Verification items for the finished model (mm, model axes). A direction names the side the tool comes from. Give positions to 0.01 mm unless a question says otherwise; leave off trailing zeros. Write each loop counter-clockwise with the first axis right and the second up, starting at its lowest first coordinate (ties: lowest second). Pieces come first, ordered by that corner, then holes. Notation, with made-up numbers: (-33.75, 31) - (24.25, 31) arc R16 cw to (24.25, 52) - close; hole circle Ø2 at (-27, 18). An arc over 180 degrees is marked (long way). Put each result on its own line as item: value.
from build123d import *

# Parameters (mm, degrees)
SKETCH2_W           = 66.5
SKETCH2_H           = 63.5
BOSS_EXTRUDE1_DEPTH = 3
SKETCH6_W           = 72
SKETCH6_H           = 69
SKETCH6_W_2         = 66.5
SKETCH6_H_2         = 63.5
BOSS_EXTRUDE2_DEPTH = 5
SKETCH14_W          = 7.5
SKETCH14_H          = 59
BOSS_EXTRUDE4_DEPTH = 14
BOSS_EXTRUDE5_DEPTH = 1.5
SKETCH16_R          = 5.5
SKETCH16_R_2        = 2.5
BOSS_EXTRUDE6_DEPTH = 2
BOSS_EXTRUDE7_DEPTH = 10
BOSS_EXTRUDE8_DEPTH = 5
SKETCH19_W          = 15
SKETCH19_H          = 7
BOSS_EXTRUDE9_DEPTH = 3


with BuildPart() as part:
    # Sketch2 → Boss-Extrude1 (new body)
    with BuildSketch(Plane(origin=(0, 0, 0), x_dir=(1, 0, 0), z_dir=(0, 1, 0))):
        Rectangle(SKETCH2_W, SKETCH2_H)
    extrude(amount=BOSS_EXTRUDE1_DEPTH)

    # Sketch6 → Boss-Extrude2 (add)
    with BuildSketch(Plane(origin=(0, 0, 0), x_dir=(1, 0, 0), z_dir=(0, 1, 0))):
        Rectangle(SKETCH6_W, SKETCH6_H)
        Rectangle(SKETCH6_W_2, SKETCH6_H_2, mode=Mode.SUBTRACT)
    extrude(amount=BOSS_EXTRUDE2_DEPTH)

    # Sketch14 → Boss-Extrude4 (add)
    with BuildSketch(Plane(origin=(0, 3, 0), x_dir=(1, 0, 0), z_dir=(0, 1, 0))):
        with Locations((-32.25, -0.25)):
            Rectangle(SKETCH14_W, SKETCH14_H)
    extrude(amount=BOSS_EXTRUDE4_DEPTH)

    # Sketch15 → Boss-Extrude5 (add)
    with BuildSketch(Plane(origin=(0, 5, 0), x_dir=(1, 0, 0), z_dir=(0, 1, 0))):
        Polygon((-34.45, 32.95), (34.45, 32.95), (34.45, -32.95), (-34.45, -32.95), (-34.45, -29.75), (-36, -29.75), (-36, -34.5), (36, -34.5), (36, 34.5), (-36, 34.5), (-36, 29.25), (-34.45, 29.25), align=None)
    extrude(amount=BOSS_EXTRUDE5_DEPTH)

    # Sketch16 → Boss-Extrude6 (add)
    # profile 1 of 4: a face of its own
    with BuildSketch(Plane.XZ):
        with Locations((-38.75, 37.25)):
            Circle(SKETCH16_R)
        with Locations(Location((-38.75, 37.25, 0), (0, 0, 270))):
            Circle(SKETCH16_R_2, mode=Mode.SUBTRACT)
    # profile 2 of 4: a face of its own
    with BuildSketch(Plane.XZ):
        with Locations((38.75, 37.25)):
            Circle(SKETCH16_R)
        with Locations(Location((38.75, 37.25, 0), (0, 0, 270))):
            Circle(SKETCH16_R_2, mode=Mode.SUBTRACT)
    # profile 3 of 4: a face of its own
    with BuildSketch(Plane.XZ):
        with Locations((38.75, -37.25)):
            Circle(SKETCH16_R)
        with Locations(Location((38.75, -37.25, 0), (0, 0, 270))):
            Circle(SKETCH16_R_2, mode=Mode.SUBTRACT)
    # profile 4 of 4: a face of its own
    with BuildSketch(Plane.XZ):
        with Locations((-38.75, -37.25)):
            Circle(SKETCH16_R)
        with Locations(Location((-38.75, -37.25, 0), (0, 0, 270))):
            Circle(SKETCH16_R_2, mode=Mode.SUBTRACT)
    extrude(amount=-BOSS_EXTRUDE6_DEPTH)

    # Sketch17 → Boss-Extrude7 (add)
    with BuildSketch(Plane.ZY.offset(24)):
        Polygon((34.5, 6.5), (33.15, 6.5), (33.15, 8.35), (32.15, 8.35), (32.15, 8.75), (33.15, 10), (34.5, 10), align=None)
    boss_extrude7 = extrude(amount=-BOSS_EXTRUDE7_DEPTH)

    # Mirror1: Boss-Extrude7 across plane
    add(boss_extrude7.mirror(Plane.XY))

    # Sketch18 → Boss-Extrude8 (add, symmetric)
    with BuildSketch(Plane.XY):
        Polygon((36, 6.5), (34.65, 6.5), (34.65, 8.45), (33.65, 8.45), (33.65, 8.85), (34.90023603, 10), (36, 10), align=None)
    extrude(amount=BOSS_EXTRUDE8_DEPTH, both=True)

    # Sketch19 → Boss-Extrude9 (add)
    with BuildSketch(Plane(origin=(0, 3, 0), x_dir=(1, 0, 0), z_dir=(0, 1, 0))):
        with Locations((15.75, -18.25)):
            Rectangle(SKETCH19_W, SKETCH19_H)
        with Locations((15.75, 0.75)):
            Rectangle(SKETCH19_W, SKETCH19_H)
    extrude(amount=BOSS_EXTRUDE9_DEPTH)


solid = part.part
Q1. Section check D-D, the plane x = 26. Record the cut outline in (y, z), plus the area to 3 significant figures.
Answers follow:
outline: (0, -34.5) - (6.5, -34.5) - (6.5, -32.95) - (5, -32.95) - (5, -31.75) - (3, -31.75) - (3, 31.75) - (5, 31.75) - (5, 32.95) - (6.5, 32.95) - (6.5, 34.5) - (0, 34.5) - close
area: 223 mm2
Q2. Release check for a two-part mould opening along Z. For faces 1 (the face through (-28.5, 10, 1)), 2 (the face through (35, 8, 5)), 3 (the face through (-39, 2, 40)) record: released by +Z, released by -Z, zero draft, split by the parting line, or undercut.
Answers follow:
face 1: undercut
face 2: released by +Z
face 3: zero draft
Q3. Section check C-C, the plane z = -6. Record the cut outline in (x, y).
Answers follow:
outline: (-36, 0) - (36, 0) - (36, 6.5) - (34.45, 6.5) - (34.45, 5) - (33.25, 5) - (33.25, 3) - (-28.5, 3) - (-28.5, 17) - (-36, 17) - close
Q4. Section check B-B, the plane x = -38.75. Record the cut outline in (y, z), plus the area to 3 significant figures.
Answers follow:
outline: (0, -42.75) - (2, -42.75) - (2, -39.75) - (0, -39.75) - close; (0, -34.75) - (2, -34.75) - (2, -31.75) - (0, -31.75) - close; (0, 31.75) - (2, 31.75) - (2, 34.75) - (0, 34.75) - close; (0, 39.75) - (2, 39.75) - (2, 42.75) - (0, 42.75) - close
area: 24.0 mm2
Q5. Set-up check for faces 4 (the face through (0, 4, 31.75)), 5 (the face through (-24, 8, 34)), 6 (the face through (-32, 17, 0)): record each of +Z, -Z, +X, -X, +Y, -Y from which the full face is reachable in a straight line by a thin tool's end or side.
Answers follow:
face 4: +Y
face 5: +Z, -Z, -X, +Y
face 6: +Z, -Z, +X, -X, +Y
Q6. Scan lines: line 1 along X through (y, z) = (1.6, 37.25); line 2 along Z through (x, y) = (16, 4); line 3 along X through (y, z) = (5.5, 14). Record each from-to range of solid material in increasing order.
Answers follow:
line 1: x = -44.25 to -41.25, -36.25 to -33.25, 33.25 to 36.25, 41.25 to 44.25
line 2: z = -34.5 to -31.75, -4.25 to 2.75, 14.75 to 21.75, 31.75 to 34.5
line 3: x = -36 to -28.5, 34.45 to 36
Q7. Go/stop test with flat-tipped pins: pin 1 Ø12 at (x, z) = (30.5, 0.5) entering from +Y; pin 2 Ø7.5 at (x, z) = (12, 19) entering from +Y; pin 3 Ø1.5 at (x, z) = (20.5, 10) entering from +Y; pin 4 Ø2 at (x, y) = (23.5, 8) entering from -Z. Record where each tip stops, or that it passes through.
Answers follow:
pin 1: stops at y = 10
pin 2: stops at y = 6
pin 3: stops at y = 3
pin 4: passes through
Q8. Section check A-A, the plane z = 37.25. Record the cut outline in (x, y).
Answers follow:
outline: (-44.25, 0) - (-41.25, 0) - (-41.25, 2) - (-44.25, 2) - close; (-36.25, 0) - (-33.25, 0) - (-33.25, 2) - (-36.25, 2) - close; (33.25, 0) - (36.25, 0) - (36.25, 2) - (33.25, 2) - close; (41.25, 0) - (44.25, 0) - (44.25, 2) - (41.25, 2) - close
